The model under review builds one solid part; all positions refer to its coordinate system, in mm. Round coordinates to 2 decimals unless told otherwise and drop trailing zeros. Order: outer loops, then holes, each group sorted by start corner. A loop starts at its lowest first (then second) coordinate and runs counter-clockwise, first axis right, second up. Notation, with made-up numbers: (-39, -19.5) - (11, -19.5) arc R17 ccw to (11, -9.5) - close; hole circle Ø11 at (48.25, 61). An arc over 180 degrees is marked (long way). One line per question, with ' | ' between items. Start each with the question number.
Item 1: Add section B-B on x = 1. State the section outline as (y, z) points (3 decimals), and give its area (3 significant figures).
Item 2: Insertion check: pin 1 Ø1.5 at (x, y) = (15.5, 18) entering from -Z. The pin has a flat end and moves straight along its axis. Give the tip position at first contact, or say it passes through.
Item 3: For L1, parallel to Y at x = 13, z = 140; L2, parallel to Y at x = -23, z = 525.5, list the stretches that pass through material, from the lowest coordinate up. Write a range as [from, to].
Item 4: Add section C-C on y = -8.5. State the section outline as (x, z) points (3 decimals).
from build123d import *

# Parameters (mm, degrees)
F1_DEPTH = 587.375
F3_DEPTH = 50.801


with BuildPart() as f1:
    # F0 (on Top) → F1 (new body)
    with BuildSketch(Plane.XY):
        with BuildLine():
            Line((22.225, 25.4), (-22.225, 25.4))
            ThreePointArc((-22.225, 25.4), (-24.470064, 24.470064), (-25.4, 22.225))
            Line((-25.4, 22.225), (-25.4, -22.225))
            ThreePointArc((-25.4, -22.225), (-24.470064, -24.470064), (-22.225, -25.4))
            Line((-22.225, -25.4), (22.225, -25.4))
            ThreePointArc((22.225, -25.4), (24.470064, -24.470064), (25.4, -22.225))
            Line((25.4, -22.225), (25.4, 22.225))
            ThreePointArc((25.4, 22.225), (24.470064, 24.470064), (22.225, 25.4))
        make_face()
        with BuildLine():
            ThreePointArc((-19.05, 17.4625), (-18.585032, 18.585032), (-17.4625, 19.05))
            Line((-17.4625, 19.05), (17.4625, 19.05))
            ThreePointArc((17.4625, 19.05), (18.585032, 18.585032), (19.05, 17.4625))
            Line((19.05, 17.4625), (19.05, -17.4625))
            ThreePointArc((19.05, -17.4625), (18.585032, -18.585032), (17.4625, -19.05))
            Line((17.4625, -19.05), (-17.4625, -19.05))
            ThreePointArc((-17.4625, -19.05), (-18.585032, -18.585032), (-19.05, -17.4625))
            Line((-19.05, -17.4625), (-19.05, 17.4625))
        make_face(mode=Mode.SUBTRACT)
    extrude(amount=F1_DEPTH)

    # F2 (on face) → F3 (cut, through all)
    with BuildSketch(Plane.YZ.offset(25.4)):
        Polygon((-25.4, 536.575), (25.4, 587.375), (-25.4, 587.375), align=None)
    extrude(amount=-F3_DEPTH, mode=Mode.SUBTRACT)


solid = f1.part
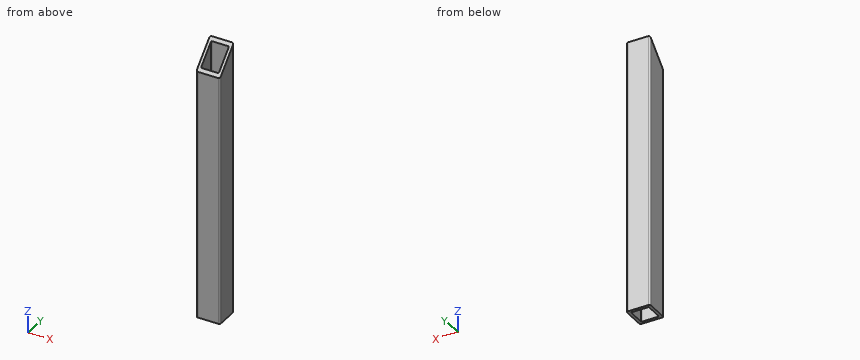
Determined:
1) outline: (-25.4, 0) - (-19.05, 0) - (-19.05, 542.925) - (-25.4, 536.575) - close; (19.05, 0) - (25.4, 0) - (25.4, 587.375) - (19.05, 581.025) - close | area: 7,140 mm2
2) pin 1: through
3) L1: [-25.4, -19.05], [19.05, 25.4] | L2: [-25.3, 25.3]
4) outline: (-25.4, 0) - (-19.05, 0) - (-19.05, 553.475) - (-25.4, 553.475) - close; (19.05, 0) - (25.4, 0) - (25.4, 553.475) - (19.05, 553.475) - close
